For this review, take the finished solid that the model builds, in its own axes (mm). Face numbers are marked on the shaded views. A direction names the side the tool comes from. Coordinates: 2 decimals unless noted, no trailing zeros. Order: outer loops, then holes, each group sorted by start corner. A loop starts at its lowest first (then second) coordinate and runs counter-clockwise, first axis right, second up. Notation, with made-up numbers: (-14.5, 37.25) -> (2.5, 37.25) arc R24 cw to (2.5, 70.25) -> close; hole circle Ø2 at (80.25, 79.25). An arc over 180 degrees is marked (long way). Answer as a JSON object with one key per item and string values. Group by question number.
1) Draft analysis for pull direction Z (two halves, no side actions). For the marked faces 3, 4 and 5, state which applies: +Z half, -Z half, draft (parallel to the pull), parting line (faces both ways), or undercut.
2) Add section D-D, the plane z = -15. Write out the cut boundary in (x, y), then the cut area to 3 significant figures.
3) Add section C-C, the plane y = 80. Write out the cut boundary in (x, z), then the cut area to 3 significant figures.
4) For pin 1 (1.5 mm diameter, centred on x = -29, z = -59.5, fed in from -Y); pin 2 (3 mm diameter, centred on x = 14.5, z = -7.5, fed in from -Y); pin 3 (8 mm diameter, centred on x = -66.5, y = -73, fed in from +Z); pin 4 (1.5 mm diameter, centred on x = -32, z = -39.5, fed in from +Y), all flat-tipped, find the tip position at first contact; note any pin that passes through.
5) Add section A-A, the plane y = 0. Write out the cut boundary in (x, z).
6) Machinability: for the marked faces 1 and 2, which of the approach directions +Z, -Z, +X, -X, +Y, -Y give a long, thin tool a straight path to every point of the face, cutting with its end or side? Answer none if there is none.
7) Wall thickness on L1, parallel to Z at x = -44, y = -32; L2, parallel to Y at x = 0, z = -28; L3, parallel to X at y = -11, z = -63.5: over which ranges is each line inside the solid? List them lowest first.
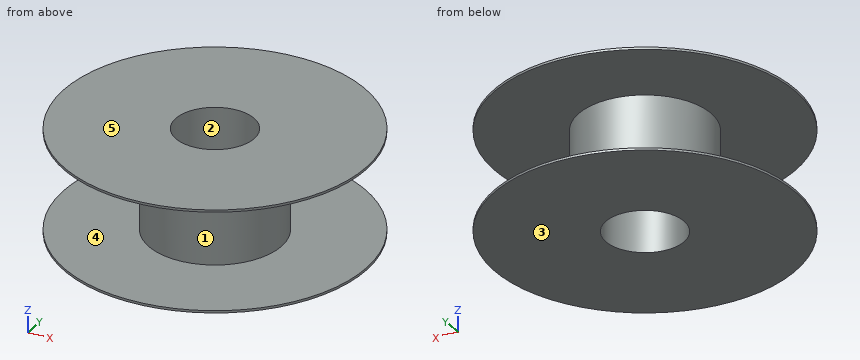
from build123d import *

# Parameters (mm, degrees)
ESBO_O1_R                = 100
ESBO_O1_R_2              = 44
ESBO_O1_R_3              = 26
RESSALTO_EXTRUS_O1_DEPTH = 1.5
ESBO_O1_3_R              = 44
ESBO_O1_3_R_2            = 26
RESSALTO_EXTRUS_O2_DEPTH = 34


with BuildPart() as part:
    # Esbo_o1 → Ressalto-extrus_o1 (new body)
    # profile 1 of 2: a face of its own
    with BuildSketch(Plane.XY):
        Circle(ESBO_O1_R)
        Circle(ESBO_O1_R_2, mode=Mode.SUBTRACT)
    # profile 2 of 2: a face of its own
    with BuildSketch(Plane.XY):
        Circle(ESBO_O1_R_2)
        Circle(ESBO_O1_R_3, mode=Mode.SUBTRACT)
    extrude(amount=-RESSALTO_EXTRUS_O1_DEPTH)

    # Esbo_o1_3 → Ressalto-extrus_o2 (add)
    with BuildSketch(Plane.XY):
        Circle(ESBO_O1_3_R)
        Circle(ESBO_O1_3_R_2, mode=Mode.SUBTRACT)
    extrude(amount=-RESSALTO_EXTRUS_O2_DEPTH)

    # Espelhar1: part across plane


with BuildPart() as part_1:
    add(part.part)
    add(part.part.mirror(Plane(origin=(0, 0, -34), x_dir=(1, 0, 0), z_dir=(0, 0, -1))))


solid = part_1.part
Output values:
{
 "1": {"face 3": "-Z half", "face 4": "undercut", "face 5": "+Z half"},
 "2": {"outline": "circle Ø88 at (0, 0); hole circle Ø52 at (0, 0)", "area": "3,960 mm²"},
 "3": {"outline": "(-60, -68) -> (60, -68) -> (60, -66.5) -> (-60, -66.5) -> close; (-60, -1.5) -> (60, -1.5) -> (60, 0) -> (-60, 0) -> close", "area": "360 mm²"},
 "4": {"pin 1": "stops at y = -33.73", "pin 2": "stops at y = -42.04", "pin 3": "stops at z = 0", "pin 4": "stops at y = 30.97"},
 "5": {"outline": "(-100, -68) -> (-26, -68) -> (-26, 0) -> (-100, 0) -> (-100, -1.5) -> (-44, -1.5) -> (-44, -66.5) -> (-100, -66.5) -> close; (26, -68) -> (100, -68) -> (100, -66.5) -> (44, -66.5) -> (44, -1.5) -> (100, -1.5) -> (100, 0) -> (26, 0) -> close"},
 "6": {"face 1": "none", "face 2": "+Z, -Z"},
 "7": {"L1": "z = -68 to -66.5, -1.5 to 0", "L2": "y = -44 to -26, 26 to 44", "L3": "x = -42.6 to -23.56, 23.56 to 42.6"}
}
